```python
from build123d import *

# Parameters (mm, degrees)
BOSS_EXTRUDE1_DEPTH        = 2.5
BOSS_EXTRUDE2_START        = -6
BOSS_EXTRUDE2_DEPTH        = 2.5
SKETCH4_W                  = 120
SKETCH4_H                  = 2.5
BOSS_EXTRUDE3_DEPTH        = 8.5
M4X0_7_TAPPED_HOLE1_D      = 3.3
SKETCH5_W                  = 30
SKETCH5_H                  = 10
BOSS_EXTRUDE4_DEPTH        = 2.5
F_4_5_4_5_DIAMETER_HOLE1_D = 4.5


with BuildPart() as part:
    # Sketch1 → Boss-Extrude1 (new body)
    with BuildSketch(Plane(origin=(0, 0, 0), x_dir=(0, 0, -1), z_dir=(1, 0, 0))):
        with BuildLine():
            Line((-60, 17.5), (-60, 0))
            Line((-60, 0), (60, 0))
            Line((60, 0), (60, 17.5))
            ThreePointArc((60, 17.5), (55.112108327, 26.094553418), (45.22673031, 26.287257619))
            ThreePointArc((45.22673031, 26.287257619), (0, 14.796523563), (-45.22673031, 26.287257619))
            ThreePointArc((-45.22673031, 26.287257619), (-55.112108327, 26.094553418), (-60, 17.5))
        make_face()
    extrude(amount=BOSS_EXTRUDE1_DEPTH)



with BuildPart() as body_2:
    # Sketch1_2 → Boss-Extrude2 (new body)
    with BuildSketch(Plane(origin=(0, 0, 0), x_dir=(0, 0, -1), z_dir=(1, 0, 0)).offset(BOSS_EXTRUDE2_START)):
        with BuildLine():
            Line((-60, 17.5), (-60, 0))
            Line((-60, 0), (60, 0))
            Line((60, 0), (60, 17.5))
            ThreePointArc((60, 17.5), (55.112108327, 26.094553418), (45.22673031, 26.287257619))
            ThreePointArc((45.22673031, 26.287257619), (0, 14.796523563), (-45.22673031, 26.287257619))
            ThreePointArc((-45.22673031, 26.287257619), (-55.112108327, 26.094553418), (-60, 17.5))
        make_face()
    extrude(amount=-BOSS_EXTRUDE2_DEPTH)


with BuildPart() as part_1:
    add(part.part)

    add(body_2.part)  # Boss-Extrude3 merges body 2
    # Sketch4 → Boss-Extrude3 (add)
    with BuildSketch(Plane.ZY):
        with Locations((0, 1.25)):
            Rectangle(SKETCH4_W, SKETCH4_H)
    extrude(amount=BOSS_EXTRUDE3_DEPTH)

    # M4x0.7 Tapped Hole1 (through all)
    with Locations(Plane(origin=(2.5, 0, 0), x_dir=(0, 0, 1), z_dir=(1, 0, 0))):
        with Locations((-50, -17.5), (50, -17.5)):
            Hole(M4X0_7_TAPPED_HOLE1_D / 2)

    # Sketch5 → Boss-Extrude4 (add)
    with BuildSketch(Plane.XZ):
        with Locations((-12.5, 40)):
            Rectangle(SKETCH5_W, SKETCH5_H)
        with Locations((-12.5, -55)):
            Rectangle(SKETCH5_W, SKETCH5_H)
        with Locations((6.5, 55)):
            Rectangle(SKETCH5_W, SKETCH5_H)
        with Locations((6.5, -40)):
            Rectangle(SKETCH5_W, SKETCH5_H)
    extrude(amount=-BOSS_EXTRUDE4_DEPTH)

    # 4.5 _4.5_ Diameter Hole1 (through all)
    with Locations(Plane(origin=(0, 2.5, 0), x_dir=(1, 0, 0), z_dir=(0, 1, 0))):
        with Locations((-22.5, 55), (16.5, 40), (16.5, -55), (-22.5, -40)):
            Hole(F_4_5_4_5_DIAMETER_HOLE1_D / 2)


solid = part_1.part
```
For this review, take the finished solid that the model builds, in its own axes (mm). A direction names the side the tool comes from. Coordinates: 2 decimals unless noted, no trailing zeros. Order: outer loops, then holes, each group sorted by start corner. A loop starts at its lowest first (then second) coordinate and runs counter-clockwise, first axis right, second up. Notation, with made-up numbers: (1.5, -39) - (5.5, -39) arc R6 cw to (5.5, -32) - close; hole circle Ø8 at (10.25, 42.5). An arc over 180 degrees is marked (long way). Answer as a JSON object with one key per item and string values. Group by question number.
1. For faces 4 (the flat face through (12, 2.5, -40)), 5 (the flat face through (12, 1, 50)), 6 (the flat face through (-18, 2.5, 40)), 7 (the flat face through (12, 1, -45)), 8 (the cylindrical face through (16.79, 1.23, -42.23)), list the 3-axis set-ups (+Z, -Z, +X, -X, +Y, -Y) from which the entire face can be reached by the end or side of a thin tool; tool diameter is ignored.
2. We need section D-D on z = -12. State the section outline as (x, y) points.
3. We need section B-B on x = -22.5. State the section outline as (y, z) points.
4. We need section A-A on y = 7.75. State the section outline as (x, z) points, then the cut area to 3 significant figures.
5. For probe 1 along Z at (x, y) = (-22.5, 0.8); probe 2 along Z at (x, y) = (16.5, 1.2); probe 3 along X at (y, z) = (0.9, -55), list the stretches that pass through material, from the lowest coordinate up.
6. We need section C-C on z = 40. State the section outline as (x, y) points, then the cut area to 3 significant figures.
7. Clearance check with flat-ended pins moving along their axes: P1, Ø2, axis at x = -19.5, y = 1, coming from the +Z side; P2, Ø8, axis at x = -16, z = 38.5, coming from the +Y side; P3, Ø5, axis at y = 15, z = -27.5, coming from the +X side. State where each tip first meets the part, or that it passes through.
8. The part is to be moulded in two halves that separate along Y. For faces 1 (the cylindrical face through (1.23, 16.11, -50.89)), 2 (the flat face through (-8.5, 11, 1)), 3 (the cylindrical face through (1.232, 26.168, 54.987)), say which applies: pulls with the +Y half, pulls with the -Y half, needs draft (parallel to the pull), parting line crosses it, or undercut.
Final values:
{
 "1": {"face 4": "+Z, -Z, +X, +Y", "face 5": "+X, +Y, -Y", "face 6": "+Z, -Z, -X, +Y", "face 7": "-Z, +X, +Y, -Y", "face 8": "+Y, -Y"},
 "2": {"outline": "(-8.5, 0) - (2.5, 0) - (2.5, 15.56) - (0, 15.56) - (0, 2.5) - (-6, 2.5) - (-6, 15.56) - (-8.5, 15.56) - close"},
 "3": {"outline": "(0, -60) - (2.5, -60) - (2.5, -57.25) - (0, -57.25) - close; (0, -52.75) - (2.5, -52.75) - (2.5, -50) - (0, -50) - close; (0, 35) - (2.5, 35) - (2.5, 37.75) - (0, 37.75) - close; (0, 42.25) - (2.5, 42.25) - (2.5, 45) - (0, 45) - close"},
 "4": {"outline": "(-8.5, -60) - (-6, -60) - (-6, 60) - (-8.5, 60) - close; (0, -60) - (2.5, -60) - (2.5, 60) - (0, 60) - close", "area": "600 mm²"},
 "5": {"probe 1": "-60 to -57.25, -52.75 to -50, 35 to 37.75, 42.25 to 45", "probe 2": "-45 to -42.25, -37.75 to -35, 50 to 52.75, 57.25 to 60", "probe 3": "-27.5 to -24.75, -20.25 to 2.5"},
 "6": {"outline": "(-27.5, 0) - (-24.75, 0) - (-24.75, 2.5) - (-27.5, 2.5) - close; (-20.25, 0) - (2.5, 0) - (2.5, 23.65) - (0, 23.65) - (0, 2.5) - (-6, 2.5) - (-6, 23.65) - (-8.5, 23.65) - (-8.5, 2.5) - (-20.25, 2.5) - close", "area": "170 mm²"},
 "7": {"P1": "z = 45", "P2": "y = 2.5", "P3": "x = 2.5"},
 "8": {"face 1": "undercut", "face 2": "needs draft", "face 3": "pulls with the +Y half"}
}
